For this review, take the finished solid that the model builds, in its own axes (mm). Round coordinates to 2 decimals unless told otherwise and drop trailing zeros. Order: outer loops, then holes, each group sorted by start corner. A loop starts at its lowest first (then second) coordinate and runs counter-clockwise, first axis right, second up. Notation, with made-up numbers: M 71.5,-21.75 L 91.5,-21.75 A30 ccw 91.5,6.25 Z; hole C -9.75,-28 d7. An arc over 180 degrees is marked long. Write item = value, one per line. Start each with the question number.
from build123d import *

# Parameters (mm, degrees)
F0_W        = 108.3307564259
F0_H        = 90.0692865252
F0_R        = 37.9662670308
F1_DEPTH    = 76.2
F2_T1_DEPTH = 159.1307564259
F2_T3_DEPTH = 140.8692865252


# Not quite as in the source:
# - a fillet or chamfer that OpenCascade refuses, or shapes differently, is made with other operations: its cross-section is extruded or revolved along the edge and cut away or added


with BuildPart() as f1:
    # F0 (on Top) → F1 (new body)
    with BuildSketch(Plane.XY):
        Rectangle(F0_W, F0_H)
        Circle(F0_R, mode=Mode.SUBTRACT)
    extrude(amount=F1_DEPTH)

    # F2: fillet of radius 10.16 on 5 edges, made by hand

    # F2_s2 → F2_t1 (cut)
    with BuildSketch(Plane.YZ.offset(-79.5653782129)):
        with BuildLine():
            ThreePointArc((-45.0346432626, 66.04), (-42.0588481595, 73.2242048969), (-34.8746432626, 76.2))
            Line((-34.8746432626, 76.2), (-45.0346432626, 76.2))
            Line((-45.0346432626, 76.2), (-45.0346432626, 66.04))
        make_face()
        with BuildLine():
            ThreePointArc((45.0346432626, 66.04), (42.0588481595, 73.2242048969), (34.8746432626, 76.2))
            Line((34.8746432626, 76.2), (45.0346432626, 76.2))
            Line((45.0346432626, 76.2), (45.0346432626, 66.04))
        make_face()
    extrude(amount=F2_T1_DEPTH, mode=Mode.SUBTRACT)

    # F2_s4 → F2_t3 (cut)
    with BuildSketch(Plane.XZ.offset(-70.4346432626)):
        with BuildLine():
            ThreePointArc((-54.1653782129, 66.04), (-51.1895831098, 73.2242048969), (-44.0053782129, 76.2))
            Line((-44.0053782129, 76.2), (-54.1653782129, 76.2))
            Line((-54.1653782129, 76.2), (-54.1653782129, 66.04))
        make_face()
        with BuildLine():
            ThreePointArc((54.1653782129, 66.04), (51.1895831098, 73.2242048969), (44.0053782129, 76.2))
            Line((44.0053782129, 76.2), (54.1653782129, 76.2))
            Line((54.1653782129, 76.2), (54.1653782129, 66.04))
        make_face()
    extrude(amount=F2_T3_DEPTH, mode=Mode.SUBTRACT)

    # F2_s5 → F2_t6 (revolve, cut)
    with BuildSketch(Plane.XZ):
        with BuildLine():
            ThreePointArc((37.9662670308, 66.04), (40.9420621339, 73.2242048969), (48.1262670308, 76.2))
            Line((48.1262670308, 76.2), (37.9662670308, 76.2))
            Line((37.9662670308, 76.2), (37.9662670308, 66.04))
        make_face()
    revolve(axis=Axis((0, 0, 76.2), (0, 0, 1)), mode=Mode.SUBTRACT)


solid = f1.part
(1) We need section B-B, the plane y = 0. Write out the cut boundary in (x, z).
(2) Draft analysis for pull direction X (two halves, no side actions). For faces 1 (the flat face through (54.165, -1, 33)), 2 (the flat face through (41, 31, 76.2)), 3 (the cylindrical face through (36.213, 11.404, 32.558)), state which applies: released by +X, released by -X, zero draft, split by the parting line, or undercut.
(3) For line 1 along Y through (x, z) = (0, 37); line 2 along X through (y, z) = (18.5, 59.5); line 3 along Y through (x, z) = (-14, 64.5), list the stretches that pass through material, from the lowest coordinate up.
(4) We need section D-D, the plane z = 68. Write out the cut boundary in (x, y), then the cut area to 3 significant figures.
(5) We need section C-C, the plane x = 0. Write out the cut boundary in (y, z).
(6) We need section A-A, the plane z = 24.5. Write out the cut boundary in (x, y), then the cut area to 3 significant figures.
Values:
q1.outline = M -54.17,0 L -37.97,0 L -37.97,66.04 A10.16 ccw -46.07,75.99 A10.16 ccw -54.17,66.04 Z; M 37.97,0 L 54.17,0 L 54.17,66.04 A10.16 ccw 46.07,75.99 A10.16 ccw 37.97,66.04 Z
q2.face_1 = released by +X
q2.face_2 = zero draft
q2.face_3 = undercut
q3.line_1 = -45.03 to -37.97, 37.97 to 45.03
q3.line_2 = -54.17 to -33.15, 33.15 to 54.17
q3.line_3 = -45.03 to -35.29, 35.29 to 45.03
q4.outline = M -53.97,-44.84 L 53.97,-44.84 L 53.97,44.84 L -53.97,44.84 Z; hole C 0,0 d76.31
q4.area = 5,110 mm²
q5.outline = M -45.03,0 L -37.97,0 L -37.97,66.04 A10.16 ccw -41.5,73.74 A10.16 ccw -45.03,66.04 Z; M 37.97,0 L 45.03,0 L 45.03,66.04 A10.16 ccw 41.5,73.74 A10.16 ccw 37.97,66.04 Z
q6.outline = M -54.17,-45.03 L 54.17,-45.03 L 54.17,45.03 L -54.17,45.03 Z; hole C 0,0 d75.93
q6.area = 5,230 mm²
